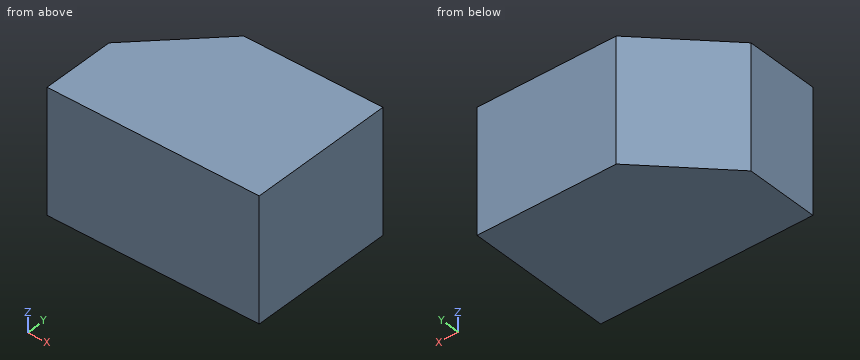
```python
from build123d import *

# Parameters (mm, degrees)
F0_W      = 43.9760684967
F0_H      = 38.9796495438
F1_DEPTH  = 145
F2_DEPTH  = 145
F3_DEPTH  = 84
F4_W      = 44.016815722
F4_H      = 37.3572036624
F5_DEPTH  = 10
F6_DEPTH  = 50
F8_DEPTH  = 50
F11_DEPTH = 84
F13_DEPTH = 45


with BuildPart() as f1:
    # F0 (on Front) → F1 (new body)
    with BuildSketch(Plane.XZ):
        with Locations((21.9880342484, 19.4898247719)):
            Rectangle(F0_W, F0_H)
    extrude(amount=F1_DEPTH)

    # F2 (add): a face of the model
    f2_faces = [f1.faces().sort_by_distance(p)[0] for p in [
        (0, -72.5, 19.4898247719),
    ]]
    extrude(f2_faces, amount=-F2_DEPTH)

    # F3 (add): a face of the model
    f3_faces = [f1.faces().sort_by_distance(p)[0] for p in [
        (72.5, -72.5, 0),
    ]]
    extrude(f3_faces, amount=-F3_DEPTH)

    # F10 (on face) → F11 (cut)
    with BuildSketch(Plane.XY.offset(84)):
        Polygon((0, -49.8955249786), (49.8742908239, 0), (0, 0), align=None)
    extrude(amount=-F11_DEPTH, mode=Mode.SUBTRACT)

    # F13 (cut): a face of the model
    f13_faces = [f1.faces().sort_by_distance(p)[0] for p in [
        (72.5, -145, 42),
    ]]
    extrude(f13_faces, amount=-F13_DEPTH, mode=Mode.SUBTRACT)


with BuildPart() as f5:
    # F4 (on face) → F5 (new body)
    with BuildSketch(Plane.XY.offset(84)):
        with Locations((22.008407861, -18.6786018312)):
            Rectangle(F4_W, F4_H)
    extrude(amount=F5_DEPTH)


with BuildPart() as f6:
    # F6 (new): a face of the model
    f6_faces = [f5.part.faces().sort_by_distance(p)[0] for p in [
        (22.008407861, 0, 89),
    ]]
    extrude(f6_faces, amount=-F6_DEPTH)


with BuildPart() as f8:
    # F8 (new): a face of the model
    f8_faces = [f6.part.faces().sort_by_distance(p)[0] for p in [
        (0, -25, 89),
    ]]
    extrude(f8_faces, amount=-F8_DEPTH)


solid = f1.part
```
The listing builds one solid part. Answer for the finished solid, in the listing's coordinates (mm). Coordinates: 2 decimals unless noted, no trailing zeros. Write each loop counter-clockwise with the first axis right and the second up, starting at its lowest first coordinate (ties: lowest second). Pieces come first, ordered by that corner, then holes. Notation, with made-up numbers: (-13, -7) - (-6, -7) arc R15 cw to (-6, 13) - close; hole circle Ø1 at (35.25, -40). An arc over 180 degrees is marked (long way). One line per item, written item: value.
1) Find section A-A (z = 47). Give the vertices of the cut face in (x, y), and give its area (3 significant figures).
Geometry check:
outline: (0, -100) - (145, -100) - (145, 0) - (49.87, 0) - (0, -49.9) - close
area: 13,300 mm2
2) Find section C-C (x = 18.5). Give the vertices of the cut face in (y, z), and give its area (3 significant figures).
Geometry check:
outline: (-100, 0) - (-31.39, 0) - (-31.39, 84) - (-100, 84) - close
area: 5,760 mm2
3) This flat-tipped pin is pushed along its axis until it touches: pin 1 Ø1 at (x, y) = (97.5, -81.5) entering from -Z. Where does it stop, or does it pass through?
Geometry check:
pin 1: stops at z = 0
4) Consider line 1 along X through (y, z) = (-38, 33.5); line 2 along X through (y, z) = (-10.5, 29.5); line 3 along Y through (x, z) = (15.5, 11). Determine where each line is inside the solid, lowest interval first. Write a range as from..to.
Geometry check:
line 1: x = 11.89..145
line 2: x = 39.38..145
line 3: y = -100..-34.39
5) Find section B-B (y = -37.5). Give the vertices of the cut face in (x, z).
Geometry check:
outline: (12.39, 0) - (145, 0) - (145, 84) - (12.39, 84) - close
